For this review, take the finished solid that the model builds, in its own axes (mm). A direction names the side the tool comes from. Give positions to 0.01 mm unless a question says otherwise; leave off trailing zeros. Loops run counter-clockwise (first coordinate to the right, second up) from the corner with the lowest first, then second, coordinate; pieces in that order, holes last. Notation, with made-up numbers: (47.5, 21) -> (61.5, 21) arc R10 cw to (61.5, 39) -> close; hole circle Ø2 at (32.5, 14). An arc over 180 degrees is marked (long way). Write each question's results on one line, items separated by ' | '. Start each with the question number.
```python
from build123d import *

# Parameters (mm, degrees)
SKETCH_1_R               = 11.8
SKETCH_1_R_2             = 17.8
EXTRUDE_2_DEPTH          = 75
CUT_EXTRUDE_1_DEPTH      = 409.99959193
CUT_EXTRUDE_1_DEPTH_BACK = 409.99959193
SKETCH_2_W               = 349.9
SKETCH_2_H               = 931.6
SKETCH_2_W_2             = 272.2
SKETCH_2_H_2             = 1939.2
FILLET_1_R               = 50


with BuildPart() as part:
    # 草图1 → 凸台-拉伸2 (new, symmetric)
    with BuildSketch(Plane.XY):
        with BuildLine():
            Line((-35.522730508, 95.251379062), (24.047591424, 34.058759041))
            ThreePointArc((24.047591424, 34.058759041), (45.036365139, 1.951247863), (52.39346962, -35.695716288))
            Line((52.39346962, -35.695716288), (52.39346962, -254.995716288))
            ThreePointArc((52.39346962, -254.995716288), (42.566387073, -303.252504348), (14.650341024, -343.823226775))
            Line((14.650341024, -343.823226775), (-33.168257533, -389.93401824))
            ThreePointArc((-33.168257533, -389.93401824), (-63.662585593, -389.379575912), (-63.108143264, -358.885247852))
            Line((-63.108143264, -358.885247852), (-3.792973322, -301.688476836))
            ThreePointArc((-3.792973322, -301.688476836), (18.829755143, -268.810595941), (26.79346962, -229.704047294))
            Line((26.79346962, -229.704047294), (26.79346962, -60.304047294))
            ThreePointArc((26.79346962, -60.304047294), (19.460018396, -22.778118982), (-1.461275938, 9.226165824))
            Line((-1.461275938, 9.226165824), (-61.03159787, 70.418785844))
            ThreePointArc((-61.03159787, 70.418785844), (-60.693460797, 95.589516134), (-35.522730508, 95.251379062))
        make_face()
        with Locations((-48.277164189, 82.835082453)):
            Circle(SKETCH_1_R, mode=Mode.SUBTRACT)
        with Locations((-48.138200399, -374.409633046)):
            Circle(SKETCH_1_R_2, mode=Mode.SUBTRACT)
    extrude(amount=EXTRUDE_2_DEPTH, both=True)

    # 草图2 → 切除-拉伸1 (cut, two sides: drawn at the far end of the back side and taken through both)
    with BuildSketch(Plane(origin=(0, 0, 0), x_dir=(0, 0, -1), z_dir=(1, 0, 0)).offset(-CUT_EXTRUDE_1_DEPTH_BACK)):
        with Locations((129.95, 450.104283712)):
            Rectangle(SKETCH_2_W, SKETCH_2_H)
        with Locations((-105.32326979, -1025.295716288)):
            Rectangle(SKETCH_2_W_2, SKETCH_2_H_2)
    extrude(amount=CUT_EXTRUDE_1_DEPTH + CUT_EXTRUDE_1_DEPTH_BACK, mode=Mode.SUBTRACT)

    # 圆角1
    fillet_1_edges = [part.edges().sort_by_distance(p)[0] for p in [
        (33.313903749, -15.695716288, 45),
        (39.5401781, -55.695716288, -30.77673021),
    ]]
    fillet(fillet_1_edges, radius=FILLET_1_R)
    fillet_1_2_edges = [part.edges().sort_by_distance(p)[0] for p in [
        (39.5401781, -55.695716288, 75),
        (33.313903749, -15.695716288, -75),
    ]]
    fillet(fillet_1_2_edges, radius=FILLET_1_R)


solid = part.part
```
1. We need section A-A (x = -13.5). Write out the cut boundary in (y, z), plus the area to 3 significant figures.
2. We need section B-B (z = -56). Write out the cut boundary in (x, y).
3. Wall thickness on L1, parallel to X at y = -369, z = -64; L2, parallel to Z at x = -28, y = -340; L3, parallel to Y at x = 45, z = 20.5: over which ranges is each line inside the solid? List them lowest first.
4. Machinability: for faces 1 (the flat face through (23, -262, -30.777)), 2 (the cylindrical face through (47.76, -5.61, 37.09)), 3 (the cylindrical face through (22.493, -31.342, 17.828)), 4 (the flat face through (-22, 60, 45)), 5 (the cylindrical face through (-63.33, -389.717, -52.579)), which of the approach directions +Z, -Z, +X, -X, +Y, -Y give a long, thin tool a straight path to every point of the face, cutting with its end or side? Answer none if there is none.
5. Draft analysis for pull direction Y (two halves, no side actions). For faces 6 (the flat face through (33, -15.696, -15)), 7 (the cylindrical face through (36.4, -40.66, 60.74)), 8 (the cylindrical face through (18.608, -269.328, -52.579)), state which applies: released by +Y, released by -Y, zero draft, split by the parting line, or undercut.
6. For pin 1 Ø2 at (x, z) = (25.5, -49.5) entering from +Y; pin 2 Ø4 at (x, z) = (-4.5, 36) entering from +Y; pin 3 Ø12 at (x, y) = (-7.5, -305) entering from -Z; pin 4 Ø22 at (y, z) = (-147, -29.5) entering from -X, all flat-tipped, find the tip position at first contact; note any pin that passes through.
7. We need section D-D (z = 54.5). Write out the cut boundary in (x, y), plus the area to 3 significant figures.
8. We need section C-C (y = -174). Write out the cut boundary in (x, z), plus the area to 3 significant figures.
Response:
1) outline: (-370.97, -75) -> (-311.05, -75) -> (-311.05, -30.78) -> (-370.97, -30.78) -> close; (21.59, 43.36) arc R50 cw to (34.3, 45) -> (72.63, 45) -> (72.63, 75) -> (21.59, 75) -> close | area: 4,190 mm2
2) outline: (-63.11, -358.89) arc R21.57 ccw to (-33.17, -389.93) -> (14.65, -343.82) arc R123.4 ccw to (52.39, -255) -> (52.39, -35.7) arc R100 ccw to (51.97, -26.47) -> (20.87, -26.47) arc R99.68 cw to (26.79, -60.3) -> (26.79, -229.7) arc R100 cw to (-3.79, -301.69) -> close; hole circle Ø35.6 at (-48.14, -374.41)
3) L1: x = -69.02 to -65.1, -31.18 to -11.46 | L2: z = -75 to -30.78 | L3: y = -55.7 to -8.7
4) face 1: +Z, +X, -X, -Y | face 2: +Z, -Z, +X, +Y | face 3: +Z, -Z, -X | face 4: -Z, +X, -X, +Y | face 5: +Z, -Z
5) face 6: released by +Y | face 7: released by -Y | face 8: undercut
6) pin 1: stops at y = -21.56 | pin 2: passes through | pin 3: stops at z = -75 | pin 4: stops at x = 26.79
7) outline: (-61.03, 70.42) -> (-1.46, 9.23) arc R99.68 cw to (25.77, -46.07) -> (52.39, -46.07) -> (52.39, -35.7) arc R100 ccw to (24.05, 34.06) -> (-35.52, 95.25) arc R17.8 ccw to start; hole circle Ø23.6 at (-48.28, 82.84) | area: 5,530 mm2
8) outline: (26.79, -75) -> (52.39, -75) -> (52.39, -30.78) -> (26.79, -30.78) -> close | area: 1,130 mm2
